Part model, mm, in its own coordinate system. Face numbers are marked on the shaded views. A direction names the side the tool comes from. Give positions to 0.01 mm unless a question says otherwise; leave off trailing zeros. Loops run counter-clockwise (first coordinate to the right, second up) from the corner with the lowest first, then second, coordinate; pieces in that order, holes last. Notation, with made-up numbers: M -37.75,62.5 L 20.25,62.5 A18 cw 20.25,76.5 Z; hole C 32.5,38.25 d11. An arc over 180 degrees is marked long. Answer in a Markdown table with one row per item.
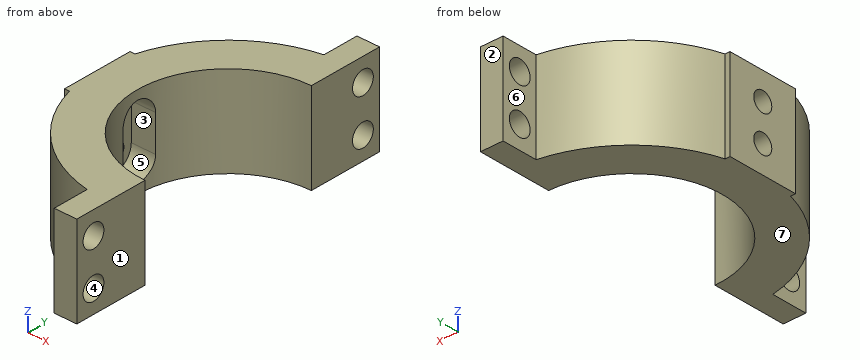
Autodesk Inventor part; units mm, degrees
ref_plane "Work Plane1" through (46.7103, 36.7, 0) normal (0, 1, 0) x (0, 0, 1)
ref_plane "Work Plane2" through (10, 0, 0) normal (0, 1, 0) x (1, 0, 0)
ref_plane "Work Plane4" through (21.3, 0, 0) normal (-1, 0, 0) x (0, -1, 0)
sketch "Sketch1" plane through (0, 0, 0) normal (0, 0, 1) x (1, 0, 0)
  arc A0 (-10, -8.75) -> (-8.75, -10) centre (-8.75, -8.75) ccw
  line L0 (-8.75, -10) -> (-3.6, -10)
  line L1 (-3.6, -10) -> (-3.1, -9.5)
  line L2 (-3.1, -9.5) -> (-3.1, -8.4)
  line L3 (-3.1, -8.4) -> (-5.5, -8.4)
  line L4 (-5.5, -8.4) -> (-5.5, -6.466)
  line L5 (-5.5, -6.466) -> (-3.134, -4.1)
  line L6 (-3.134, -4.1) -> (3.134, -4.1)
  line L7 (3.134, -4.1) -> (5.5, -6.466)
  line L8 (5.5, -6.466) -> (5.5, -8.4)
  line L9 (5.5, -8.4) -> (3.1, -8.4)
  line L10 (3.1, -8.4) -> (3.1, -9.5)
  line L11 (3.1, -9.5) -> (3.6, -10)
  line L12 (3.6, -10) -> (8.75, -10)
  arc A1 (8.75, -10) -> (10, -8.75) centre (8.75, -8.75) ccw
  line L13 (10, -8.75) -> (10, -3.6)
  line L14 (10, -3.6) -> (9.5, -3.1)
  line L15 (9.5, -3.1) -> (8.4, -3.1)
  line L16 (8.4, -3.1) -> (8.4, -5.5)
  line L17 (8.4, -5.5) -> (6.466, -5.5)
  line L18 (6.466, -5.5) -> (4.1, -3.134)
  line L19 (4.1, -3.134) -> (4.1, 3.134)
  line L20 (4.1, 3.134) -> (6.466, 5.5)
  line L21 (6.466, 5.5) -> (8.4, 5.5)
  line L22 (8.4, 5.5) -> (8.4, 3.1)
  line L23 (8.4, 3.1) -> (9.5, 3.1)
  line L24 (9.5, 3.1) -> (10, 3.6)
  line L25 (10, 3.6) -> (10, 8.75)
  arc A2 (10, 8.75) -> (8.75, 10) centre (8.75, 8.75) ccw
  line L26 (8.75, 10) -> (3.6, 10)
  line L27 (3.6, 10) -> (3.1, 9.5)
  line L28 (3.1, 9.5) -> (3.1, 8.4)
  line L29 (3.1, 8.4) -> (5.5, 8.4)
  line L30 (5.5, 8.4) -> (5.5, 6.466)
  line L31 (5.5, 6.466) -> (3.134, 4.1)
  line L32 (3.134, 4.1) -> (-3.134, 4.1)
  line L33 (-3.134, 4.1) -> (-5.5, 6.466)
  line L34 (-5.5, 6.466) -> (-5.5, 8.4)
  line L35 (-5.5, 8.4) -> (-3.1, 8.4)
  line L36 (-3.1, 8.4) -> (-3.1, 9.5)
  line L37 (-3.1, 9.5) -> (-3.6, 10)
  line L38 (-3.6, 10) -> (-8.75, 10)
  arc A3 (-8.75, 10) -> (-10, 8.75) centre (-8.75, 8.75) ccw
  line L39 (-10, 8.75) -> (-10, 3.6)
  line L40 (-10, 3.6) -> (-9.5, 3.1)
  line L41 (-9.5, 3.1) -> (-8.4, 3.1)
  line L42 (-8.4, 3.1) -> (-8.4, 5.5)
  line L43 (-8.4, 5.5) -> (-6.466, 5.5)
  line L44 (-6.466, 5.5) -> (-4.1, 3.134)
  line L45 (-4.1, 3.134) -> (-4.1, -3.134)
  line L46 (-4.1, -3.134) -> (-6.466, -5.5)
  line L47 (-6.466, -5.5) -> (-8.4, -5.5)
  line L48 (-8.4, -5.5) -> (-8.4, -3.1)
  line L49 (-8.4, -3.1) -> (-9.5, -3.1)
  line L50 (-9.5, -3.1) -> (-10, -3.6)
  line L51 (-10, -3.6) -> (-10, -8.75)
  circle A4 centre (0, 0) radius 2.5
  circle A5 centre (46.7, 0) radius 4.5
  arc A6 (46.7103, 25.4) -> (46.7103, -25.4) centre (46.7, 0) ccw
  line L52 (10, 10) -> (16.35, 10)
  line L53 (16.35, 10) -> (16.35, -10)
  line L54 (16.35, -10) -> (10, -10)
  line L55 (10, -10) -> (10, 10)
  arc A7 (46.7103, 36.7) -> (46.7103, -36.7) centre (46.7, 0) ccw
  line L56 (46.7103, 36.7) -> (46.7103, 25.4)
  line L57 (46.7103, -25.4) -> (46.7103, -36.7)
  dimension "d0" = 50.8
  dimension "d1" = 20
  dimension "d2" = 6.35
extrude "Extrusion1" add sketch "Sketch1" along normal blind 25.4 contours L13 L55 A7 L54 | L55 L25 L52 A7 | A7 L52 L53 L54 | L54 L53 L52 A7 L56 A6 L57
ref_plane "Work Plane1" through (46.7103, 36.7, 0) normal (0, 1, 0) x (0, 0, 1)
sketch "Sketch2" plane through (46.7103, 36.7, 0) normal (0, 1, 0) x (0, 0, 1)
  line L0 (0, 0) -> (25.4, 0)
  line L1 (25.4, -35.3216) -> (25.4, 0)
  line L2 (0, 0) -> (25.4, 0)
  line L3 (25.4, 0) -> (25.4, -6.35)
  line L4 (25.4, -6.35) -> (0, -6.35)
  line L5 (0, -6.35) -> (0, 0)
  point P0 (0, -46.7103)
  dimension "d6" = 6.35
extrude "Extrusion2" add sketch "Sketch2" along normal mid plane 19.05
ref_plane "Work Plane2" through (10, 0, 0) normal (0, 1, 0) x (1, 0, 0)
mirror "Mirror1" about plane through (10, 0, 0) normal (0, 1, 0) of "Extrusion2"
sketch "Sketch3" plane through (46.7103, -25.4, 25.4) normal (1, 0, 0) x (0, 0, -1)
  circle A0 centre (19.05, -15.7382) radius 3.175
  circle A1 centre (6.35, -15.7382) radius 3.175
  circle A2 centre (6.35, 66.5382) radius 3.175
  circle A3 centre (19.05, 66.5382) radius 3.175
  point P0 (25.4, 25.4)
extrude "Extrusion3" cut sketch "Sketch3" against normal through all
ref_plane "Work Plane4" through (21.3, 0, 0) normal (-1, 0, 0) x (0, -1, 0)
ref_plane "Work Plane3" through (72.1, 0, 0) normal (-1, 0, 0) x (0, -1, 0)
sketch "Sketch4" plane through (72.1, 0, 0) normal (-1, 0, 0) x (0, -1, 0)
  line L0 (0, 0) -> (0, 25.4) construction
  line L1 (-10, 25.4) -> (10, 25.4)
  circle A0 centre (0, 17.78) radius 2.75
  circle A1 centre (0, 7.62) radius 2.75
  line L2 (-25.4, 0) -> (25.4, 0)
  dimension "d13" = 5.5
  dimension "d14" = 7.62
  dimension "d15" = 7.62
extrude "Extrusion4" cut sketch "Sketch4" along normal through all
sketch "Sketch5" plane through (72.1, 0, 0) normal (-1, 0, 0) x (0, -1, 0)
  spline S0 degree 2 poles (2.75, 17.78) (2.75, 13.0169) (-1.375, 15.3984) (-5.5, 17.78) (-1.375, 20.1616) (2.75, 22.5431) (2.75, 17.78) knots 0 0 0 0.333333 0.333333 0.666667 0.666667 1 1 1 weights 1 0.5 1 0.5 1 0.5 1
  spline S1 degree 2 poles (2.75, 7.62) (2.75, 2.8569) (-1.375, 5.2384) (-5.5, 7.62) (-1.375, 10.0016) (2.75, 12.3831) (2.75, 7.62) knots 0 0 0 0.333333 0.333333 0.666667 0.666667 1 1 1 weights 1 0.5 1 0.5 1 0.5 1
  circle A0 centre (0, 7.62) radius 2.75
  line L0 (5, 12.7) -> (5, 7.62)
  arc A1 (-5, 7.62) -> (5, 7.62) centre (0, 7.62) ccw
  spline S2 degree 7 poles (2.75, 17.78) (2.75, 18.0802) (2.7118, 18.38) (2.6355, 18.6767) (2.52, 18.9674) (2.3634, 19.248) (2.1631, 19.5126) (1.7177, 19.9454) (1.4837, 20.1274) (1.2158, 20.2864) (0.9183, 20.4129) (0.5978, 20.4988) (0.2624, 20.5386) (-0.4242, 20.519) (-0.7584, 20.4587) (-1.0728, 20.3535) (-1.3607, 20.2102) (-1.617, 20.0371) (-1.8389, 19.8434) (-2.2394, 19.407) (-2.4132, 19.1552) (-2.5494, 18.8907) (-2.6501, 18.6181) (-2.7166, 18.3405) (-2.75, 18.0604) (-2.75, 17.4798) (-2.7118, 17.18) (-2.6355, 16.8833) (-2.52, 16.5926) (-2.3634, 16.312) (-2.1631, 16.0474) (-1.7177, 15.6146) (-1.4837, 15.4326) (-1.2158, 15.2736) (-0.9183, 15.1471) (-0.5978, 15.0612) (-0.2624, 15.0214) (0.4242, 15.041) (0.7584, 15.1013) (1.0728, 15.2065) (1.3607, 15.3498) (1.617, 15.5229) (1.8389, 15.7166) (2.2394, 16.153) (2.4132, 16.4048) (2.5494, 16.6693) (2.6501, 16.9419) (2.7166, 17.2195) (2.75, 17.4996) (2.75, 17.78) knots 0 0 0 0 0 0 0 0 0.14065 0.14065 0.14065 0.14065 0.14065 0.14065 0.254122 0.254122 0.254122 0.254122 0.254122 0.254122 0.369156 0.369156 0.369156 0.369156 0.369156 0.369156 0.500342 0.500342 0.500342 0.500342 0.500342 0.500342 0.640802 0.640802 0.640802 0.640802 0.640802 0.640802 0.754121 0.754121 0.754121 0.754121 0.754121 0.754121 0.869 0.869 0.869 0.869 0.869 0.869 1 1 1 1 1 1 1 1
  line L1 (25.4, 0) -> (-25.4, 0)
  line L2 (-25.4, 0) -> (-25.4, 25.4)
  line L3 (25.4, 25.4) -> (-25.4, 25.4)
  line L4 (25.4, 0) -> (25.4, 25.4)
  line L5 (-10, 25.4) -> (10, 25.4)
  line L6 (0, 25.4) -> (0, 20.53)
  line L7 (0, 15.03) -> (0, 10.37) construction
  line L8 (0, 4.87) -> (0, 0)
  line L9 (-5.6857, 12.7) -> (9.2801, 12.7) construction
  line L10 (-5, 7.62) -> (-5, 12.7)
  line L11 (5, 12.7) -> (5, 17.78)
  arc A2 (5, 17.78) -> (-5, 17.78) centre (0, 17.78) ccw
  line L12 (-5, 17.78) -> (-5, 12.7)
extrude "Extrusion5" cut sketch "Sketch5" along normal blind 57.15 contours L0 A1 L10 L12 A2 L11
properties part number "DremelHolder"
(1) Pull direction Y, two halves, no side cores. Call the marked faces 1, 2, 3 and 4: +Y half, -Y half, draft (parallel to the pull), parting line (faces both ways), or undercut.
Recorded:
| item | result |
|---|---|
| face 1 | draft |
| face 2 | +Y half |
| face 3 | undercut |
| face 4 | undercut |
(2) Saw through at D-D (z = 6). Write the cut outline in (x, y) (3 decimals), plus the area to 3 significant figures.
Recorded:
| item | result |
|---|---|
| outline | M 10,-10 L 11.389,-10 A36.7 ccw 40.36,-36.148 L 40.36,-37.983 L 46.71,-37.983 L 46.71,-25.4 A25.4 cw 21.744,-4.73 L 14.95,-4.73 L 14.95,-2.222 L 10,-2.222 Z; M 10,2.222 L 14.95,2.222 L 14.95,4.73 L 21.744,4.73 A25.4 cw 46.71,25.4 L 46.71,37.983 L 40.36,37.983 L 40.36,36.148 A36.7 ccw 11.389,10 L 10,10 Z; M 40.36,-46.225 L 46.71,-46.225 L 46.71,-44.294 L 40.36,-44.294 Z; M 40.36,44.294 L 46.71,44.294 L 46.71,46.225 L 40.36,46.225 Z |
| area | 1,070 mm^2 |
(3) Which spindle directions (+Z, -Z, +X, -X, +Y, -Y) get a long thin tool onto all of the face, cutting with end or side? Do the marked faces 5, 6 and 7. Say none if no direction does.
Recorded:
| item | result |
|---|---|
| face 5 | +X |
| face 6 | +Z, -Z, -X, +Y |
| face 7 | -Z, +X, -X, +Y, -Y |
(4) Saw through at A-A (z = 13.25). Write the cut outline in (x, y) (3 decimals), plus the area to 3 significant figures.
Recorded:
| item | result |
|---|---|
| outline | M 10,-10 L 11.389,-10 A36.7 ccw 40.36,-36.148 L 40.36,-46.225 L 46.71,-46.225 L 46.71,-25.4 A25.4 cw 21.797,-5 L 14.95,-5 L 14.95,5 L 21.797,5 A25.4 cw 46.71,25.4 L 46.71,46.225 L 40.36,46.225 L 40.36,36.148 A36.7 ccw 11.389,10 L 10,10 Z |
| area | 1,170 mm^2 |
(5) Saw through at B-B (y = 0). Write the cut outline in (x, z), plus the area to 3 significant figures.
Recorded:
| item | result |
|---|---|
| outline | M 10,0 L 21.3,0 L 21.3,2.62 L 14.95,2.62 L 14.95,4.87 L 10,4.87 Z; M 10,10.37 L 14.95,10.37 L 14.95,15.03 L 10,15.03 Z; M 10,20.53 L 14.95,20.53 L 14.95,22.78 L 21.3,22.78 L 21.3,25.4 L 10,25.4 Z |
| area | 105 mm^2 |
(6) Drill centre lines: line 1 along Z through (x, y) = (12.7, 0); line 2 along Y through (x, z) = (44.25, 19.05) (3 decimals); line 3 along X through (y, z) = (-2, 21.5). Where is each one in solid material? Low to high.
Recorded:
| item | result |
|---|---|
| line 1 | z = 0 to 4.87, 10.37 to 15.03, 20.53 to 25.4 |
| line 2 | y = -46.225 to -44.313, -37.963 to -25.282, 25.282 to 37.963, 44.313 to 46.225 |
| line 3 | x = 10 to 14.95 |
(7) Pin check, flat tips, straight feed: pin 1 Ø3.5 at (x, z) = (19.5, 10.5) entering from -Y; pin 2 Ø8 at (y, z) = (25, 7.5) entering from +X; pin 3 Ø7.5 at (y, z) = (41.14, 19.05) entering from -X; pin 4 Ø3 at (y, z) = (8, 18.5) entering from +X. Stop position of each tip, or through.
Recorded:
| item | result |
|---|---|
| pin 1 | stops at y = -26.44 |
| pin 2 | stops at x = 46.71 |
| pin 3 | stops at x = 40.36 |
| pin 4 | stops at x = 23.14 |
(8) Saw through at C-C (x = 18). Write the cut outline in (y, z).
Recorded:
| item | result |
|---|---|
| outline | M -22.87,0 L 22.87,0 L 22.87,25.4 L -22.87,25.4 Z; hole M -5,7.62 A5 ccw 5,7.62 L 5,17.78 A5 ccw -5,17.78 Z |
